Autodesk Inventor part; units mm, degrees
ref_plane "YZ-Ebene" through (0, 0, 0) normal (1, 0, 0) x (0, 1, 0)
ref_plane "XZ-Ebene" through (0, 0, 0) normal (0, 1, 0) x (-1, 0, 0)
ref_plane "XY-Ebene" through (0, 0, 0) normal (0, 0, 1) x (1, 0, 0)
sketch "Skizze1" plane through (0, 0, 0) normal (0, 0, 1) x (1, 0, 0)
  line L0 (-2.1971, 0) -> (10.2828, 0)
  line L1 (0, -2.7828) -> (0, 16.6971)
  line L2 (0, 5) -> (1.2, 5)
  line L3 (1.2, 5) -> (1.2, 2.75)
  line L4 (1.2, 2.75) -> (5.2, 2.75)
  arc A0 (6.4, 3.95) -> (5.2, 2.75) centre (6.4, 2.75) ccw
  line L5 (6.4, 3.95) -> (7.6, 3.95)
  line L6 (7.6, 3.95) -> (7.6, 8.75)
  line L7 (7.6, 8.75) -> (8.5, 8.75)
  line L8 (8.5, 8.75) -> (8.5, 13.5)
  line L9 (8.5, 13.5) -> (2, 13.5)
  arc A1 (2, 13.5) -> (0, 11.5) centre (2, 11.5) ccw
  line L10 (0, 11.5) -> (0, 5)
  point P0 (0, 0)
  dimension "d6" = 2.75
  dimension "d7" = 5
  dimension "d8" = 8.75
  dimension "d9" = 13.5
  dimension "d10" = 1.2
  dimension "d11" = 2.4
  dimension "d12" = 0.9
  dimension "d13" = 1.2
  dimension "d14" = 2
  dimension "d15" = 8.5
revolve "Umdrehung1" add sketch "Skizze1" angle 360 about axis through (-10, 0, 0) along (1, 0, 0)
sketch "Skizze2" plane through (0, 0, 0) normal (-1, 0, 0) x (0, 0, 1)
  circle A0 centre (0, 0) radius 5
  line L0 (-18.9, 0) -> (18.9, 0)
  circle A1 centre (0, 0) radius 5
  circle A2 centre (0, 0) radius 11.5
  point P0 (10.5, 0)
  dimension "d18" = 10.5
hole "Bohrung1" at (0, 0, 10.5) direction (1, 0, 0) diameter 3 end through all counterbore diameter 5.5 counterbore depth 3
pattern_circular "Runde Anordnung1" count 4 over 360 about axis through (3.2, 0, 0) along (-1, 0, 0) of "Bohrung1"
thread "Gewinde1"
properties part number "Zylinderkopf_ra8846s" material "Stahl, Guss"
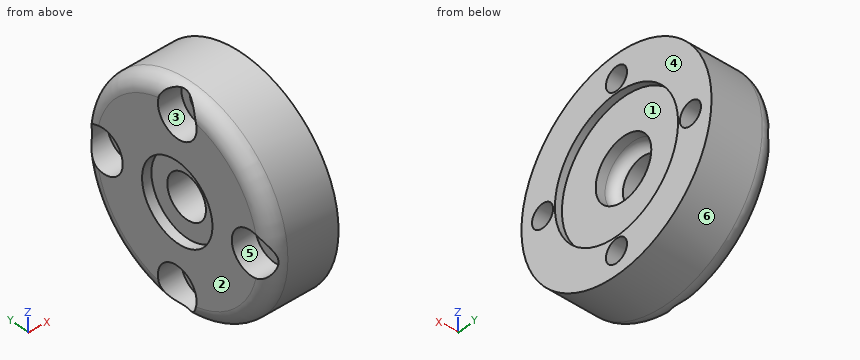
Check sheet for the modelled part. Datum: model origin and axes. Units: mm. Face numbers are marked on the shaded views. A direction names the side the tool comes from. Round coordinates to 2 decimals unless told otherwise and drop trailing zeros. Loops run counter-clockwise (first coordinate to the right, second up) from the corner with the lowest first, then second, coordinate; pieces in that order, holes last. Notation, with made-up numbers: (5, 60) -> (58, 60) arc R20 ccw to (58, 94) -> close; hole circle Ø11 at (68, -15). An arc over 180 degrees is marked (long way). Answer in a Markdown table with one row per item.
Q1. Thickness scan on L1, parallel to X at y = -3.25, z = -3.25; L2, parallel to X at y = 11.25, z = -2.25; L3, parallel to Y at x = 2.75, z = 12.25. Record the ranges inside material, lowest first.
Data:
| item | result |
|---|---|
| L1 | x = 1.2 to 7.6 |
| L2 | x = 3 to 8.5 |
| L3 | y = -5.67 to -2.12, 2.12 to 5.67 |
Q2. Set-up check for the marked faces 1, 2 and 3: record each of +Z, -Z, +X, -X, +Y, -Y from which the full face is reachable in a straight line by a thin tool's end or side.
Data:
| item | result |
|---|---|
| face 1 | +X |
| face 2 | +Z, -Z, -X, +Y, -Y |
| face 3 | -X |
Q3. Sectioned sample at A-A on x = 4. Enter the section's corners in (y, z), then the cut area to 3 significant figures.
Data:
| item | result |
|---|---|
| outline | circle Ø27 at (0, 0); hole circle Ø3 at (-10.5, 0); hole circle Ø5.5 at (0, 0); hole circle Ø3 at (0, -10.5); hole circle Ø3 at (0, 10.5); hole circle Ø3 at (10.5, 0) |
| area | 521 mm^2 |
Q4. Sectioned sample at B-B on z = 0. Give the number of separate pieces and of enclosed holes in the cut face, then the cut area to 3 significant figures.
Data:
| item | result |
|---|---|
| separate pieces | 4 |
| enclosed holes | 0 |
| area | 94.7 mm^2 |
Q5. Release check for a two-part mould opening along Z. For the marked faces 4, 5 and 6 record: released by +Z, released by -Z, zero draft, split by the parting line, or undercut.
Data:
| item | result |
|---|---|
| face 4 | zero draft |
| face 5 | undercut |
| face 6 | split by the parting line |
Q6. Go/stop test with flat-tipped pins: P1, Ø2, axis at x = 5.5, z = -2.5, coming from the -Y side; P2, Ø3, axis at x = 5, y = -4.5, coming from the -Z side; P3, Ø1.6, axis at y = 10, z = -1.5, coming from the -X side. Record where each tip stops, or that it passes through.
Data:
| item | result |
|---|---|
| P1 | stops at y = -13.42 |
| P2 | stops at z = -13.16 |
| P3 | stops at x = 3 |
Q7. Sectioned sample at C-C on x = 6. Enter the section's corners in (y, z), then the cut area to 3 significant figures.
Data:
| item | result |
|---|---|
| outline | circle Ø27 at (0, 0); hole circle Ø3 at (-10.5, 0); hole circle Ø7.76 at (0, 0); hole circle Ø3 at (0, -10.5); hole circle Ø3 at (0, 10.5); hole circle Ø3 at (10.5, 0) |
| area | 497 mm^2 |
